```python
from build123d import *

# Parameters (mm, degrees)
F1_DEPTH = 125
F3_R     = 10
F4_T     = -2.5


# Not quite as in the source:
# - a shell that OpenCascade refuses in one call is made with other operations: the cavity is built on its own and cut out


with BuildPart() as f1:
    # F0 (on Front) → F1 (new body)
    with BuildSketch(Plane.XZ):
        Polygon((206.0437292722, 62.0864819473), (6.2040649354, 35.4162448123), (6.2040649354, -174.5837551877), (166.2040649354, -174.5837551877), align=None)
    extrude(amount=F1_DEPTH)

    # F2: F1 across plane


with BuildPart() as f1_1:
    add(f1.part)
    add(f1.part.mirror(Plane.XZ))

    # F3
    f3_edges = [f1_1.edges().sort_by_distance(p)[0] for p in [
        (106.123897, -125, 48.751363),
        (206.043729, 0, 62.086482),
        (186.123897, -125, -56.248637),
        (6.204065, -125, -69.583755),
        (86.204065, -125, -174.583755),
        (166.204065, 0, -174.583755),
        (106.123897, 125, 48.751363),
        (6.204065, 0, 35.416245),
        (186.123897, 125, -56.248637),
        (6.204065, 125, -69.583755),
        (86.204065, 125, -174.583755),
        (6.204065, 0, -174.583755),
    ]]
    fillet(f3_edges, radius=F3_R)

    # F4: a shell. OpenCascade refuses it in one call, so the cavity is built on its own and cut out:
    # the body offset inwards by the wall thickness, plus a prism from it out through each open face.
    f4_core = offset(f1_1.part, amount=F4_T, mode=Mode.PRIVATE)
    f4_exits = [f4_core.faces().sort_by_distance(p)[0] for p in [
        (104.076238, 0, 45.955921),
    ]]
    add(f4_core, mode=Mode.SUBTRACT)
    extrude(f4_exits, amount=-F4_T, mode=Mode.SUBTRACT)


solid = f1_1.part
```
Model file for the job. Use its own axes, mm. A direction names the side the tool comes from. Round coordinates to 2 decimals unless told otherwise and drop trailing zeros. Write each loop counter-clockwise with the first axis right and the second up, starting at its lowest first coordinate (ties: lowest second). Pieces come first, ordered by that corner, then holes. Notation, with made-up numbers: (68.25, 44.25) - (103.25, 44.25) arc R6 cw to (103.25, 54.25) - close; hole circle Ø1 at (63, -3). An arc over 180 degrees is marked (long way). Use CSV: the item, a comma, the result in double quotes. Start each with the question number.
Item 1: Band-saw the part on A-A (y = -64.5). Write the cut outline in (x, z).
Item 2: Drill centre lines: L1, parallel to Y at x = 29, z = -112.5; L2, parallel to Z at x = 140.5, y = 18.5; L3, parallel to X at y = -70.5, z = -47. Where is each one in solid material? Low to high. Write a range as [from, to].
Item 3: Tool access for faces 1 (the face through (10.959, -1.61, -169.945)), 2 (the face through (185.448, -1.61, -60.266)): list every direction of +Z, -Z, +X, -X, +Y, -Y with a clear straight run to the whole face (end or side of a thin tool).
Item 4: Two-plate mould, pull along Z, no slides. Class faces 3 (the face through (87.966, 121.993, -171.732)), 4 (the face through (9.21, -122.15, -70.3)), 5 (the face through (87.97, -120.24, -169.95)): released by +Z, released by -Z, zero draft, split by the parting line, or undercut.
Item 5: Pin check, flat tips, straight feed: P1, Ø13, axis at x = 105, z = 49, coming from the -Y side; P2, Ø6, axis at x = 126.5, y = -8, coming from the +Z side; P3, Ø10, axis at y = -36, z = -94, coming from the +X side. Stop position of each tip, or through.
Checked values:
1,outline,"(6.2, -164.58) arc R10 ccw to (16.2, -174.58) - (157.75, -174.58) arc R10 ccw to (167.61, -166.24) - (203.79, 48.72) arc R10 ccw to (192.61, 60.29) - (192.94, 57.82) arc R7.5 cw to (201.33, 49.14) - (165.14, -165.83) arc R7.5 cw to (157.75, -172.08) - (16.2, -172.08) arc R7.5 cw to (8.7, -164.58) - (8.7, 26.66) arc R7.5 cw to (15.21, 34.1) - (14.88, 36.57) arc R10 ccw to (6.2, 26.66) - close"
2,L1,"y = [-125, -122.5], [122.5, 125]"
2,L2,"z = [-174.58, -172.08]"
2,L3,"x = [6.2, 8.7], [185.15, 187.68]"
3,face 1,"none"
3,face 2,"-Z, +X, +Y, -Y"
4,face 3,"released by -Z"
4,face 4,"zero draft"
4,face 5,"undercut"
5,P1,"stops at y = -124.21"
5,P2,"stops at z = -172.08"
5,P3,"stops at x = 180.61"
